from build123d import *

# Parameters (mm, degrees)
ESQUISSE1_R        = 8
BOSS_EXTRU_3_DEPTH = 10


with BuildPart() as part:
    # Esquisse1 → Boss.-Extru.3 (new body)
    with BuildSketch(Plane(origin=(0, 0, 0), x_dir=(1, 0, 0), z_dir=(0, 1, 0))):
        with BuildLine():
            Line((-198.535533906, 140.467889787), (-140.467889787, 198.535533906))
            ThreePointArc((-140.467889787, 198.535533906), (-138.845773043, 199.619397663), (-136.932355881, 200))
            Line((-136.932355881, 200), (-108.642059072, 200))
            ThreePointArc((-108.642059072, 200), (-106.728641911, 199.619397663), (-105.106525166, 198.535533906))
            Line((-105.106525166, 198.535533906), (-86.822253919, 180.251262659))
            ThreePointArc((-86.822253919, 180.251262659), (-85.200137175, 179.167398902), (-83.286720013, 178.786796564))
            Line((-83.286720013, 178.786796564), (80.808477816, 178.786796564))
            ThreePointArc((80.808477816, 178.786796564), (82.721894978, 179.167398902), (84.344011722, 180.251262659))
            Line((84.344011722, 180.251262659), (102.628282969, 198.535533906))
            ThreePointArc((102.628282969, 198.535533906), (104.250399713, 199.619397663), (106.163816875, 200))
            Line((106.163816875, 200), (134.922487193, 200))
            ThreePointArc((134.922487193, 200), (136.805633434, 199.631820402), (138.411445264, 198.581504094))
            Line((138.411445264, 198.581504094), (198.488958072, 140.056393487))
            ThreePointArc((198.488958072, 140.056393487), (199.606777092, 138.418495531), (200, 136.474889393))
            Line((200, 136.474889393), (200, 108.642059072))
            ThreePointArc((200, 108.642059072), (199.619397663, 106.728641911), (198.535533906, 105.106525167))
            Line((198.535533906, 105.106525167), (180.251262658, 86.822253919))
            ThreePointArc((180.251262658, 86.822253919), (179.167398902, 85.200137175), (178.786796564, 83.286720013))
            Line((178.786796564, 83.286720013), (178.786796564, -83.293766644))
            ThreePointArc((178.786796564, -83.293766644), (179.165099385, -85.201622818), (180.242762637, -86.820780044))
            Line((180.242762637, -86.820780044), (198.544033927, -105.210368915))
            ThreePointArc((198.544033927, -105.210368915), (199.621697179, -106.82952614), (200, -108.737382314))
            Line((200, -108.737382314), (200, -136.645047547))
            ThreePointArc((200, -136.645047547), (199.621697179, -138.552903722), (198.544033927, -140.172060947))
            Line((198.544033927, -140.172060947), (140.469336148, -198.5270134))
            ThreePointArc((140.469336148, -198.5270134), (138.844277599, -199.617091455), (136.925302221, -200))
            Line((136.925302221, -200), (108.737382314, -200))
            ThreePointArc((108.737382314, -200), (106.82952614, -199.621697179), (105.210368915, -198.544033927))
            Line((105.210368915, -198.544033927), (86.820780044, -180.242762637))
            ThreePointArc((86.820780044, -180.242762637), (85.201622818, -179.165099385), (83.293766644, -178.786796564))
            Line((83.293766644, -178.786796564), (-83.286720013, -178.786796564))
            ThreePointArc((-83.286720013, -178.786796564), (-85.200137175, -179.167398902), (-86.822253919, -180.251262658))
            Line((-86.822253919, -180.251262658), (-105.106525166, -198.535533906))
            ThreePointArc((-105.106525166, -198.535533906), (-106.728641911, -199.619397663), (-108.642059072, -200))
            Line((-108.642059072, -200), (-136.932355881, -200))
            ThreePointArc((-136.932355881, -200), (-138.845773043, -199.619397663), (-140.467889787, -198.535533906))
            Line((-140.467889787, -198.535533906), (-198.535533906, -140.467889787))
            ThreePointArc((-198.535533906, -140.467889787), (-199.619397663, -138.845773043), (-200, -136.932355881))
            Line((-200, -136.932355881), (-200, -108.642059072))
            ThreePointArc((-200, -108.642059072), (-199.619397663, -106.728641911), (-198.535533906, -105.106525166))
            Line((-198.535533906, -105.106525166), (-180.251262658, -86.822253919))
            ThreePointArc((-180.251262658, -86.822253919), (-179.167398902, -85.200137175), (-178.786796564, -83.286720013))
            Line((-178.786796564, -83.286720013), (-178.786796564, 83.286720013))
            ThreePointArc((-178.786796564, 83.286720013), (-179.167398902, 85.200137175), (-180.251262658, 86.822253919))
            Line((-180.251262658, 86.822253919), (-198.535533906, 105.106525166))
            ThreePointArc((-198.535533906, 105.106525166), (-199.619397663, 106.728641911), (-200, 108.642059072))
            Line((-200, 108.642059072), (-200, 136.932355881))
            ThreePointArc((-200, 136.932355881), (-199.619397663, 138.845773043), (-198.535533906, 140.467889787))
        make_face()
        with Locations(Location((120.524036122, -178.786796564, 0), (0, 0, 270))):  # turned: the seam where the file's is
            Circle(ESQUISSE1_R, mode=Mode.SUBTRACT)
        with Locations(Location((-178.786796564, -120.524036122, 0), (0, 0, 270))):  # turned: the seam where the file's is
            Circle(ESQUISSE1_R, mode=Mode.SUBTRACT)
        with Locations(Location((-120.524036122, 178.786796564, 0), (0, 0, 270))):  # turned: the seam where the file's is
            Circle(ESQUISSE1_R, mode=Mode.SUBTRACT)
        with Locations(Location((178.786796564, 120.524036122, 0), (0, 0, 270))):  # turned: the seam where the file's is
            Circle(ESQUISSE1_R, mode=Mode.SUBTRACT)
        with Locations(Location((-178.786796564, 120.524036122, 0), (0, 0, 90))):  # turned: the seam where the file's is
            Circle(ESQUISSE1_R, mode=Mode.SUBTRACT)
        with Locations(Location((120.524036122, 178.786796564, 0), (0, 0, 90))):  # turned: the seam where the file's is
            Circle(ESQUISSE1_R, mode=Mode.SUBTRACT)
        with Locations(Location((178.786796564, -120.524036122, 0), (0, 0, 90))):  # turned: the seam where the file's is
            Circle(ESQUISSE1_R, mode=Mode.SUBTRACT)
        with Locations(Location((-120.524036122, -178.786796564, 0), (0, 0, 90))):  # turned: the seam where the file's is
            Circle(ESQUISSE1_R, mode=Mode.SUBTRACT)
    extrude(amount=-BOSS_EXTRU_3_DEPTH)


solid = part.part
Model file for the job. Use its own axes, mm. A direction names the side the tool comes from. Give positions to 0.01 mm unless a question says otherwise; leave off trailing zeros. Loops run counter-clockwise (first coordinate to the right, second up) from the corner with the lowest first, then second, coordinate; pieces in that order, holes last. Notation, with made-up numbers: (-11, -1.5) -> (5, -1.5) arc R32 ccw to (5, 27.5) -> close; hole circle Ø2 at (-38, -30). An arc over 180 degrees is marked (long way). Use a Markdown table: item, result. Add a question column.
(1) Mould opens along Z. For faces 1 (the flat face through (-96.09, -4.93, -189.52)), 2 (the cylindrical face through (-117.46, -4.93, 171.397)), 3 (the flat face through (-189.52, -4.93, 96.09)), 4 (the flat face through (-123, -5, 200)) say: +Z half, -Z half, draft (parallel to the pull), parting line (faces both ways), or undercut.
(2) Drop flat-ended pins along their axis: pin 1 Ø1.5 at (y, z) = (-6.5, -89.5) entering from +X; pin 2 Ø13 at (x, z) = (-120.52, 178.79) entering from -Y; pin 3 Ø4 at (y, z) = (-6.5, 90.5) entering from -X; pin 4 Ø6 at (y, z) = (-5, -37.5) entering from +X. Give the stop position or say it passes through.
(3) Slice it at D-D on y = -5.5. Give the number of separate pieces and of enclosed holes in the cut face, and give its area (3 significant figures).
(4) Tool access for faces 5 (the flat face through (-178.787, -5, 1)), 6 (the flat face through (189.52, -4.93, -96.09)), 7 (the flat face through (168.03, -4.93, -169.73)): list every direction of +Z, -Z, +X, -X, +Y, -Y with a clear straight run to the whole face (end or side of a thin tool).
(5) Wall check: line 1 along Z through (x, y) = (180.5, -2); line 2 along X through (y, z) = (-8, 121); line 3 along Z through (x, y) = (-45.5, -6.25). Give the ranges that are in metal, low to high.
(6) Slice it at A-A on z = -122.5. List the corners of the cut face in (x, y).
(7) Slice it at B-B on x = 27. List the corners of the cut face in (y, z), and give its area (3 significant figures).
(8) Slice it at C-C on z = 59. List the corners of the cut face in (x, y).
Filled sheet:
| question | item | result |
|---|---|---|
| 1 | face 1 | -Z half |
| 1 | face 2 | undercut |
| 1 | face 3 | undercut |
| 1 | face 4 | +Z half |
| 2 | pin 1 | x = 183.68 |
| 2 | pin 2 | through |
| 2 | pin 3 | x = -185.93 |
| 2 | pin 4 | x = 178.79 |
| 3 | separate pieces | 1 |
| 3 | enclosed holes | 8 |
| 3 | area | 135,000 mm2 |
| 4 | face 5 | -X, +Y, -Y |
| 4 | face 6 | +X, +Y, -Y |
| 4 | face 7 | -Z, +X, +Y, -Y |
| 5 | line 1 | -157.58 to -128.34, -112.71 to -87.07, 87.08 to 112.71, 128.34 to 158.3 |
| 5 | line 2 | -200 to -186.77, -170.8 to 170.8, 186.77 to 200 |
| 5 | line 3 | -178.79 to 178.79 |
| 6 | outline | (-200, -10) -> (-186.54, -10) -> (-186.54, 0) -> (-200, 0) -> close; (-171.03, -10) -> (171.03, -10) -> (171.03, 0) -> (-171.03, 0) -> close; (186.54, -10) -> (200, -10) -> (200, 0) -> (186.54, 0) -> close |
| 7 | outline | (-10, -178.79) -> (0, -178.79) -> (0, 178.79) -> (-10, 178.79) -> close |
| 7 | area | 3,580 mm2 |
| 8 | outline | (-178.79, -10) -> (178.79, -10) -> (178.79, 0) -> (-178.79, 0) -> close |
